Build history of the part. All positions in model axes, mm. A direction names the side the tool comes from. Round coordinates to 2 decimals unless told otherwise and drop trailing zeros. Write each loop counter-clockwise with the first axis right and the second up, starting at its lowest first coordinate (ties: lowest second). Pieces come first, ordered by that corner, then holes. Notation, with made-up numbers: M 22,-4.5 L 26,-4.5 A17 ccw 26,22.5 Z; hole C -33,-16.5 d9. An arc over 180 degrees is marked long. Write item = value, one per line.
from build123d import *

# Parameters (mm, degrees)
SKETCH1_W           = 100
SKETCH1_H           = 60
BOSS_EXTRUDE1_DEPTH = 10
SKETCH2_R           = 2.5
CUT_EXTRUDE1_DEPTH  = 60.160797831
SKETCH3_R           = 16
CUT_EXTRUDE2_DEPTH  = 7
SKETCH4_R           = 12.5
CUT_EXTRUDE3_DEPTH  = 59.72818744
SKETCH5_R           = 1.5
CUT_EXTRUDE4_DEPTH  = 60.160797831
SKETCH6_R           = 3.25
CUT_EXTRUDE5_DEPTH  = 4
CIRPATTERN1_COUNT   = 4


with BuildPart() as part:
    # Sketch1 → Boss-Extrude1 (new body)
    with BuildSketch(Plane(origin=(0, 0, 0), x_dir=(1, 0, 0), z_dir=(0, 1, 0))):
        Rectangle(SKETCH1_W, SKETCH1_H)
    extrude(amount=BOSS_EXTRUDE1_DEPTH)

    # Sketch2 → Cut-Extrude1 (cut, through all)
    with BuildSketch(Plane(origin=(0, 10, 0), x_dir=(1, 0, 0), z_dir=(0, 1, 0))):
        with Locations(Location((-45, -20, 0), (0, 0, 270))):
            Circle(SKETCH2_R)
        with Locations(Location((-45, 0, 0), (0, 0, 270))):
            Circle(SKETCH2_R)
        with Locations(Location((-45, 20, 0), (0, 0, 270))):
            Circle(SKETCH2_R)
    cut_extrude1 = extrude(amount=-CUT_EXTRUDE1_DEPTH, mode=Mode.SUBTRACT)

    # Mirror1: Cut-Extrude1 across plane
    add(cut_extrude1.mirror(Plane(origin=(0, 0, 0), x_dir=(0, 0, 1), z_dir=(1, 0, 0))), mode=Mode.SUBTRACT)

    # Sketch3 → Cut-Extrude2 (cut)
    with BuildSketch(Plane(origin=(0, 10, 0), x_dir=(1, 0, 0), z_dir=(0, 1, 0))):
        with Locations(Location((0, 0, 0), (0, 0, 270))):
            Circle(SKETCH3_R)
    extrude(amount=-CUT_EXTRUDE2_DEPTH, mode=Mode.SUBTRACT)

    # Sketch4 → Cut-Extrude3 (cut, through all)
    with BuildSketch(Plane(origin=(0, 3, 0), x_dir=(1, 0, 0), z_dir=(0, 1, 0))):
        with Locations(Location((0, 0, 0), (0, 0, 270))):
            Circle(SKETCH4_R)
    extrude(amount=-CUT_EXTRUDE3_DEPTH, mode=Mode.SUBTRACT)

    # Sketch5 → Cut-Extrude4 (cut, through all)
    with BuildSketch(Plane(origin=(0, 10, 0), x_dir=(1, 0, 0), z_dir=(0, 1, 0))):
        with Locations(Location((-21, 21, 0), (0, 0, 270))):
            Circle(SKETCH5_R)
    cut_extrude4 = extrude(amount=-CUT_EXTRUDE4_DEPTH, mode=Mode.SUBTRACT)

    # Sketch6 → Cut-Extrude5 (cut)
    with BuildSketch(Plane(origin=(0, 10, 0), x_dir=(1, 0, 0), z_dir=(0, 1, 0))):
        with Locations(Location((-21, 21, 0), (0, 0, 270))):
            Circle(SKETCH6_R)
    cut_extrude5 = extrude(amount=-CUT_EXTRUDE5_DEPTH, mode=Mode.SUBTRACT)

    # CirPattern1: Cut-Extrude4, Cut-Extrude5 ×4 about axis
    cirpattern1_axis = Axis((0, 0, 0), (0, 1, 0))
    add([cut_extrude4.rotate(cirpattern1_axis, i * 360 / CIRPATTERN1_COUNT) for i in range(1, CIRPATTERN1_COUNT)], mode=Mode.SUBTRACT)
    add([cut_extrude5.rotate(cirpattern1_axis, i * 360 / CIRPATTERN1_COUNT) for i in range(1, CIRPATTERN1_COUNT)], mode=Mode.SUBTRACT)


solid = part.part
1. Band-saw the part on C-C (y = 4.5). Count the separate pieces of the cut face and the enclosed holes in it, plus the area to 3 significant figures.
Responses:
separate_pieces = 1
enclosed_holes = 11
area = 5,050 mm²
2. Band-saw the part on B-B (x = 45). List the corners of the cut face in (y, z), plus the area to 3 significant figures.
Responses:
outline = M 0,-30 L 10,-30 L 10,-22.5 L 0,-22.5 Z; M 0,-17.5 L 10,-17.5 L 10,-2.5 L 0,-2.5 Z; M 0,2.5 L 10,2.5 L 10,17.5 L 0,17.5 Z; M 0,22.5 L 10,22.5 L 10,30 L 0,30 Z
area = 450 mm²
3. Mould opens along X. For faces 3 (the face through (-1, 5, 30)), 4 (the face through (-50, 5, 0)), 5 (the face through (-8, 3, -10)), 6 (the face through (50, 5, 0)) say: pulls with the +X half, pulls with the -X half, needs draft (parallel to the pull), parting line crosses it, or undercut.
Responses:
face_3 = needs draft
face_4 = pulls with the -X half
face_5 = undercut
face_6 = pulls with the +X half
4. Band-saw the part on D-D (z = -10.5). List the corners of the cut face in (x, y).
Responses:
outline = M -50,0 L -6.78,0 L -6.78,3 L -12.07,3 L -12.07,10 L -50,10 Z; M 6.78,0 L 50,0 L 50,10 L 12.07,10 L 12.07,3 L 6.78,3 Z
5. Band-saw the part on A-A (x = 0). List the corners of the cut face in (y, z), plus the area to 3 significant figures.
Responses:
outline = M 0,-30 L 10,-30 L 10,-16 L 3,-16 L 3,-12.5 L 0,-12.5 Z; M 0,12.5 L 3,12.5 L 3,16 L 10,16 L 10,30 L 0,30 Z
area = 301 mm²
6. Probe probe 1 along Z at (x, y) = (21, 7.2); probe 2 along Z at (x, y) = (21, 2.3); probe 3 along X at (y, z) = (7.05, 21). List the from-to ranges inside material, lowest first.
Responses:
probe_1 = -30 to -24.25, -17.75 to 17.75, 24.25 to 30
probe_2 = -30 to -22.5, -19.5 to 19.5, 22.5 to 30
probe_3 = -50 to -47.29, -42.71 to -24.25, -17.75 to 17.75, 24.25 to 42.71, 47.29 to 50
7. Tool access for faces 1 (the face through (-46.5, 5.1, -22)), 2 (the face through (20.857, 8.028, 24.247)): list every direction of +Z, -Z, +X, -X, +Y, -Y with a clear straight run to the whole face (end or side of a thin tool).
Responses:
face_1 = +Y, -Y
face_2 = +Y
8. Flat gauge pins, fed straight in: pin 1 (4.5 mm diameter, centred on x = 45, z = 0, fed in from -Y); pin 2 (5 mm diameter, centred on x = -21, z = -21, fed in from +Y). Where does each tip first touch, or does it go through?
Responses:
pin_1 = through
pin_2 = 6
